Check sheet for the modelled part. Datum: model origin and axes. Units: mm. Face numbers are marked on the shaded views. Round coordinates to 2 decimals unless told otherwise and drop trailing zeros. Write each loop counter-clockwise with the first axis right and the second up, starting at its lowest first coordinate (ties: lowest second). Pieces come first, ordered by that corner, then holes. Notation, with made-up numbers: M 2.25,43 L 13.25,43 A26 cw 13.25,72 Z; hole C 0,43 d10. An arc over 180 degrees is marked long. Put each result on its own line as item: value.
Autodesk Inventor part; units mm, degrees
ref_plane "YZ Plane" through (0, 0, 0) normal (1, 0, 0) x (0, 1, 0)
ref_plane "XZ Plane" through (0, 0, 0) normal (0, 1, 0) x (-1, 0, 0)
ref_plane "XY Plane" through (0, 0, 0) normal (0, 0, 1) x (1, 0, 0)
sketch "スケッチ1" plane through (0, 0, 0) normal (0, 0, 1) x (1, 0, 0)
  circle A0 centre (0, 0) radius 2
  dimension "d13" = 4
extrude "押し出し1" add sketch "スケッチ1" along normal blind 10
sketch "スケッチ2" plane through (0, 0, 10) normal (0, 0, 1) x (1, 0, 0)
  point P0 (0, 0)
  point P1 (0, 0)
hole "穴1" at (0, 0, 10) direction (0, 0, -1) diameter 1.567 end through all
chamfer "面取り1" distance 0.2 angle 45 4 edges at (0, 0.7835, 10) (0, 0.7835, 0) (-2, 0, 10) (-2, 0, 0)
properties part number "ARU-2010" material "鋼、炭素鋼"
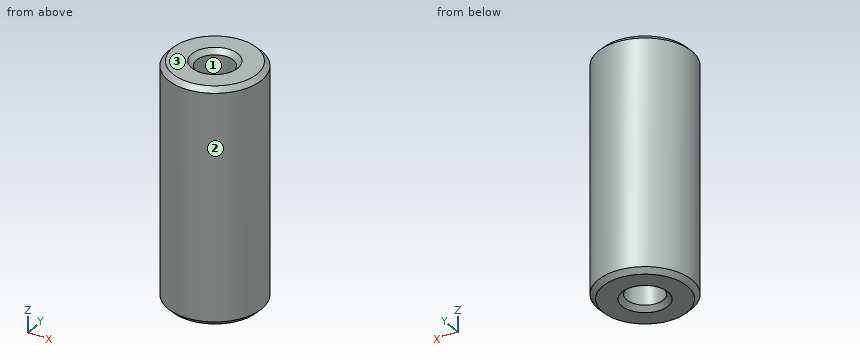
1. Cross-section at C-C (z = 1). Enter the section's corners in (x, y), then the cut area to 3 significant figures.
Computed values:
outline: C 0,0 d4; hole C 0,0 d1.57
area: 10.6 mm2
2. Release check for a two-part mould opening along X. For the marked faces 1, 2 and 3 record: +X half, -X half, draft (parallel to the pull), parting line (faces both ways), or undercut.
Computed values:
face 1: undercut
face 2: parting line
face 3: draft
3. Cross-section at A-A (x = 0). Enter the section's corners in (y, z).
Computed values:
outline: M -2,0.2 L -1.8,0 L -0.98,0 L -0.78,0.2 L -0.78,9.8 L -0.98,10 L -1.8,10 L -2,9.8 Z; M 0.78,0.2 L 0.98,0 L 1.8,0 L 2,0.2 L 2,9.8 L 1.8,10 L 0.98,10 L 0.78,9.8 Z
4. Scan lines: probe 1 along Y at (x, z) = (0, 5); probe 2 along Y at (x, z) = (-0.35, 4.75). Record each from-to range of solid material in increasing order.
Computed values:
probe 1: y = -2 to -0.78, 0.78 to 2
probe 2: y = -1.97 to -0.7, 0.7 to 1.97
5. Depth check by flat-ended pin: pin 1 Ø1.3 at (x, y) = (0, 0) entering from -Z; pin 2 Ø1.5 at (x, z) = (1.5, 8) entering from -Y. Enter the tip coordinate at first touch or a pass-through.
Computed values:
pin 1: passes through
pin 2: stops at y = -1.85
